Here's how the part is built. I have some questions about the finished solid (model axes, mm). A direction names the side the tool comes from. Give positions to 0.01 mm unless a question says otherwise; leave off trailing zeros. Write each question's results on one line, items separated by ' | '. Start each with the question number.
Q1. I'm going to push flat-ended pins straight in: pin 1 (8 mm diameter, centred on x = 7.5, z = -0.5, fed in from +Y); pin 2 (5 mm diameter, centred on y = 12, z = 17.5, fed in from +X); pin 3 (5 mm diameter, centred on x = 13.5, y = 8.5, fed in from -Z). Where does each tip first touch, or does it pass through?
Q2. For faces 5 (the face through (18, 80.005, 0)), 6 (the face through (4.51, 71.17, 14.31)), which set-ups out of +Z, -Z, +X, -X, +Y, -Y let a thin tool reach every point of the face, with its end or its side?
Q3. Thinking about a two-plate mould opening in Y: for faces 1 (the face through (-15, 78.505, -6)), 2 (the face through (15.497, 70.714, -3.441)), 3 (the face through (15, 80.005, 4)), 4 (the face through (19.2, 0.005, 17.3)), which applies, pulls with the +Y half, pulls with the -Y half, needs draft (parallel to the pull), parting line crosses it, or undercut?
Q4. I need wall thicknesses on line 1 along Z through (x, y) = (0, 79.75); line 2 along Z through (x, y) = (0, 79); line 3 along X through (y, z) = (75, 0) (3 decimals). Which ranges of each line are inside material? Lowest first, please. Write a range as [from, to].
Autodesk Inventor part; units mm, degrees
sketch "CD Nozzle Sketch" plane through (0, 0, 0) normal (1, 0, 0) x (0, 1, 0)
  line L0 (15.0042, -20) -> (15.0042, -1.5)
  line L1 (15.875, -1.5) -> (15.875, -20)
  arc A0 (6.35, -34.925) -> (15.875, -20) centre (-26.9286, -3.185) ccw
  line L2 (15.875, -1.5) -> (20.0042, -1.5)
  line L3 (20.0042, -1.5) -> (20.0042, 0)
  arc A1 (25.5095, -80) -> (5, -35) centre (-81.2197, -101.4697) ccw
  arc A2 (26.0708, -80) -> (6.35, -34.925) centre (-90.9256, -104.3355) ccw
  arc A3 (5, -35) -> (15.0042, -20) centre (-26.6763, -3.0373) ccw
  line L4 (16.5042, 0) -> (16.5042, -0.75)
  line L5 (16.5042, -0.75) -> (17.5042, -0.75)
  line L6 (17.5042, -0.75) -> (17.5042, 0)
  line L7 (17.5042, 0) -> (20.0042, 0)
  line L8 (0, 1) -> (0, 0)
  line L9 (0, 1) -> (0, 0)
  line L10 (0, 3.175) -> (0, 0)
  line L11 (0, -0.75) -> (0, 0)
  line L12 (26.0708, -80) -> (25.5095, -80)
  line L13 (15.0042, -1.5) -> (15.0042, 0)
  line L14 (15.0042, 0) -> (16.5042, 0)
  line L15 (0, 0) -> (0, -80)
  dimension "d34" = 45
  dimension "d39" = 35
revolve "CD Nozzle" add sketch "CD Nozzle Sketch" angle 360 about axis through (0, 0, 0) along (0, 0, -1)
fillet "Fillet14" radius 15 1 edges at (0, -15.875, -20)
fillet "Fillet15" radius 10 1 edges at (0, -6.35, -34.925)
fillet "Fillet16" radius 10 1 edges at (0, -5, -35)
fillet "Fillet17" radius 10 1 edges at (0, -15.0042, -20)
move or copy body "Move Body1" bodies to move or copy 1 copy no rotation origin (0, 0, 0) rotation axis (0, 0, 1) rotation angle -90
move or copy body "Move Body2" bodies to move or copy 1 copy no rotation origin (0, 0, 0) rotation axis (0, 0, 1) rotation angle -90
move or copy body "Move Body3" bodies to move or copy 1 copy no rotation origin (0, 0, 0) rotation axis (1, 0, 0) rotation angle -90
move or copy body "Move Body4" bodies to move or copy 1 copy no translate (0, 79.375, 0)
move or copy body "Move Body5" bodies to move or copy 1 copy no translate (0, 0.63, 0)
properties part number "alpha-i" material "Steel, Mild"
Geometry check:
1) pin 1: y = 53.17 | pin 2: x = 17.56 | pin 3: z = -21.52
2) face 5: +Z, -Z, +X, -X, +Y | face 6: +Y
3) face 1: undercut | face 2: undercut | face 3: pulls with the +Y half | face 4: pulls with the -Y half
4) line 1: [-20, -17.5], [-16.5, -15], [15, 16.5], [17.5, 20] | line 2: [-20, -15], [15, 20] | line 3: [-15.875, -15.004], [15.004, 15.875]
